Job drawing, mm, ordinate dimensions from the low corner. One solid piece. Coordinates: 2 decimals unless noted, no trailing zeros. Order: outer loops, then holes, each group sorted by start corner. A loop starts at its lowest first (then second) coordinate and runs counter-clockwise, first axis right, second up. Notation, with made-up numbers: (-40, 77) -> (-9, 77) arc R10 ccw to (-9, 95) -> close; hole circle Ø4 at (-31, 21). An arc over 180 degrees is marked (long way). Use CSV: the item, a comma, the result in double quotes. Start each with the question number.
(1) Cut at B-B on y = 180. Write the cut outline in (x, z).
(2) Cut at A-A on x = 100. Write the cut outline in (y, z), plus the area to 3 significant figures.
(3) Probe L1, parallel to X at y = 179, z = 0.2; L2, parallel to Y at x = 100, z = 0.7. List the from-to ranges inside material, lowest first.
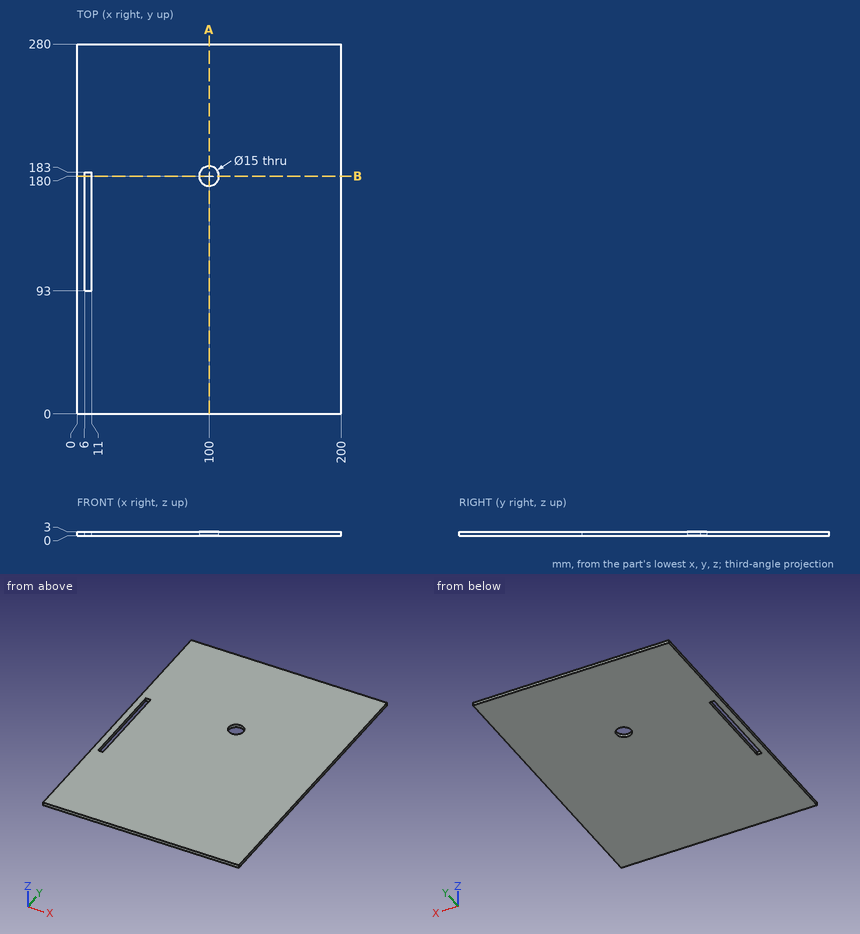
Outcome:
1,outline,"(0, 0) -> (6, 0) -> (6, 3) -> (0, 3) -> close; (11, 0) -> (92.5, 0) -> (92.5, 3) -> (11, 3) -> close; (107.5, 0) -> (200, 0) -> (200, 3) -> (107.5, 3) -> close"
2,outline,"(0, 0) -> (172.5, 0) -> (172.5, 3) -> (0, 3) -> close; (187.5, 0) -> (280, 0) -> (280, 3) -> (187.5, 3) -> close"
2,area,"795 mm2"
3,L1,"0 to 6, 11 to 92.57, 107.43 to 200"
3,L2,"0 to 172.5, 187.5 to 280"
